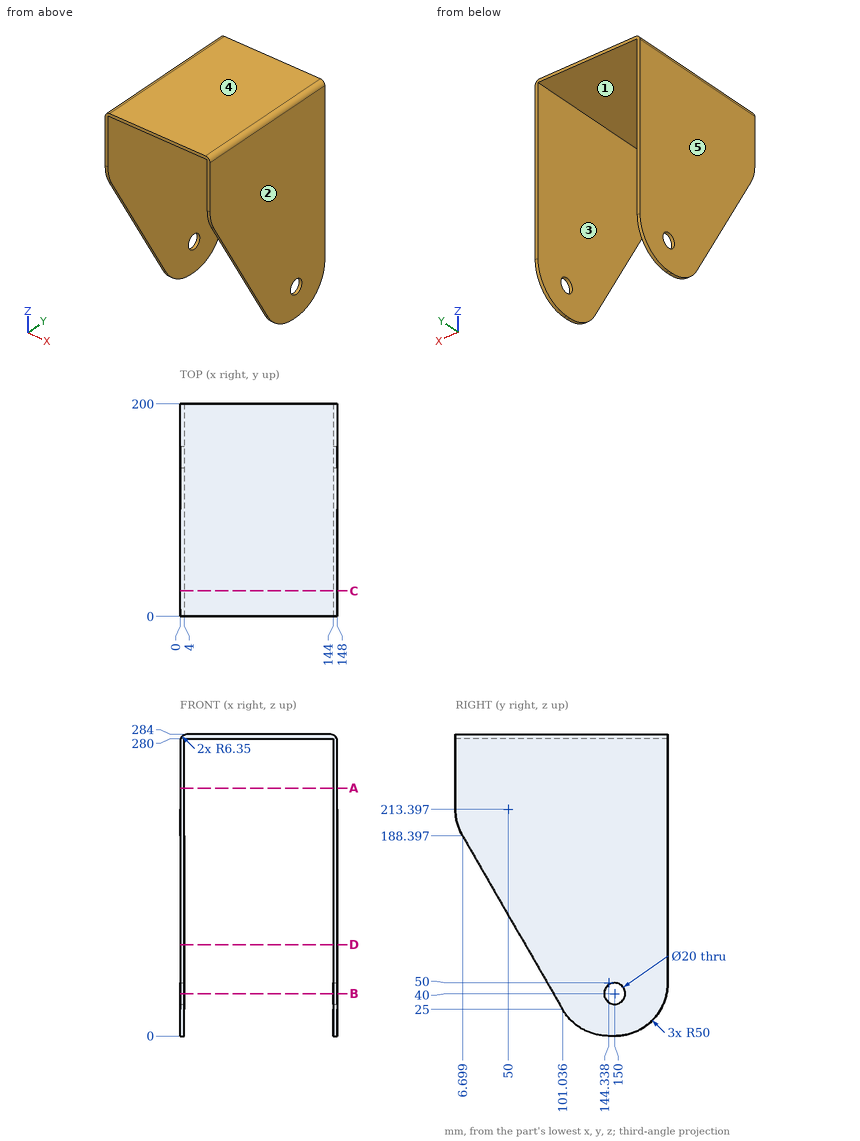
Part print with two shaded views. Sizes in mm from the minimum x, y, z corner. A direction names the side the tool comes from. Round coordinates to 2 decimals unless told otherwise and drop trailing zeros. Write each loop counter-clockwise with the first axis right and the second up, starting at its lowest first coordinate (ties: lowest second). Pieces come first, ordered by that corner, then holes. Notation, with made-up numbers: M 1.25,21 L 26.25,21 A31 cw 26.25,60 Z; hole C 28.5,44 d1. An arc over 180 degrees is marked long. Answer as CSV lines item,"result". Start each with the question number.
1) Mould opens along X. For the marked faces 3, 4 and 5 say: +X half, -X half, draft (parallel to the pull), parting line (faces both ways), or undercut.
2) Band-saw the part on D-D (z = 86). List the corners of the cut face in (x, y).
3) Drop a flat-ended pin along its axis: pin 1 (2 mm diameter, centred on x = 20, y = 176.5, fed in from -Z). Give the stop position or say it passes through.
4) Band-saw the part on B-B (z = 40). List the corners of the cut face in (x, y), then the cut area to 3 significant figures.
5) Which spindle directions (+Z, -Z, +X, -X, +Y, -Y) get a long thin tool onto all of the face, cutting with end or side? Do the marked faces 1 and 2. Say none if no direction does.
6) Drill centre lines: L1, parallel to X at y = 172.5, z = 60; L2, parallel to Z at x = 19, y = 32; L3, parallel to Z at x = 147, y = 150. Where is each one in solid material? Low to high.
7) Band-saw the part on A-A (z = 233.5). List the corners of the cut face in (x, y).
8) Band-saw the part on C-C (y = 24). List the corners of the cut face in (x, z).
Worked out:
1,face 3,"undercut"
1,face 4,"draft"
1,face 5,"-X half"
2,outline,"M 0,65.82 L 4,65.82 L 4,200 L 0,200 Z; M 144,65.82 L 148,65.82 L 148,200 L 144,200 Z"
3,pin 1,"z = 280"
4,outline,"M 0,92.38 L 4,92.38 L 4,140 L 0,140 Z; M 0,160 L 4,160 L 4,198.99 L 0,198.99 Z; M 144,92.38 L 148,92.38 L 148,140 L 144,140 Z; M 144,160 L 148,160 L 148,198.99 L 144,198.99 Z"
4,area,"693 mm²"
5,face 1,"-Z, +Y, -Y"
5,face 2,"+Z, -Z, +X, +Y, -Y"
6,L1,"0 to 4, 144 to 148"
6,L2,"280 to 284"
6,L3,"0 to 30, 50 to 281.07"
7,outline,"M 0,0 L 4,0 L 4,200 L 0,200 Z; M 144,0 L 148,0 L 148,200 L 144,200 Z"
8,outline,"M 0,158.43 L 4,158.43 L 4,280 L 144,280 L 144,158.43 L 148,158.43 L 148,277.65 A6.35 ccw 141.65,284 L 6.35,284 A6.35 ccw 0,277.65 Z"
